Autodesk Inventor part; units mm, degrees
ref_plane "YZ Plane" through (0, 0, 0) normal (1, 0, 0) x (0, 1, 0)
ref_plane "XZ Plane" through (0, 0, 0) normal (0, 1, 0) x (-1, 0, 0)
ref_plane "XY Plane" through (0, 0, 0) normal (0, 0, 1) x (1, 0, 0)
sketch "Sketch1" plane through (0, 0, 0) normal (0, 0, 1) x (1, 0, 0)
  circle A0 centre (0, 0) radius 3.9624
  dimension "cap_diam" = 7.9248
extrude "Extrusion1" add sketch "Sketch1" along normal blind 4.826
sketch "Sketch2" plane through (0, 0, 0) normal (0, 0, -1) x (-1, 0, 0)
  circle A0 centre (0, 0) radius 3.9624
  circle A1 centre (0, 0) radius 2.413
  dimension "thread_diam" = 4.826
extrude "Extrusion2" add sketch "Sketch2" along normal blind 31.75 contours A1
thread "Thread1"
chamfer "Chamfer1" distance 0.4064 angle 45 1 edges at (2.413, 0, -31.75)
chamfer "Chamfer2" distance 0.635 angle 45 1 edges at (-3.9624, 0, 4.826)
sketch "Sketch4" plane through (0, 0, 4.826) normal (0, 0, 1) x (1, 0, 0)
  circle A0 centre (0, 0) radius 3.3274
  circle A1 centre (0, 0) radius 1.9844
  dimension "d21" = 3.9688
extrude "Extrusion4" cut sketch "Sketch4" against normal blind 0.3048 contours A1
chamfer "Chamfer3" distance 0.3048 angle 45 1 edges at (-1.9844, 0, 4.826)
sketch "Sketch5" plane through (0, 0, 4.826) normal (0, 0, 1) x (1, 0, 0)
  circle A0 centre (0, 0) radius 2.2892 construction
  line L0 (0, 2.2914) -> (1.9844, 1.1457)
  line L1 (1.9844, 1.1457) -> (1.9844, -1.1457)
  line L2 (1.9844, -1.1457) -> (0, -2.2914)
  line L3 (0, -2.2914) -> (-1.9844, -1.1457)
  line L4 (-1.9844, -1.1457) -> (-1.9844, 1.1457)
  line L5 (-1.9844, 1.1457) -> (0, 2.2914)
  dimension "d27" = 3.9688
extrude "Extrusion5" cut sketch "Sketch5" against normal blind 2.9718
equation "\"d21\" = hex_diam"
properties part number "10-32 x1000" material "Steel"
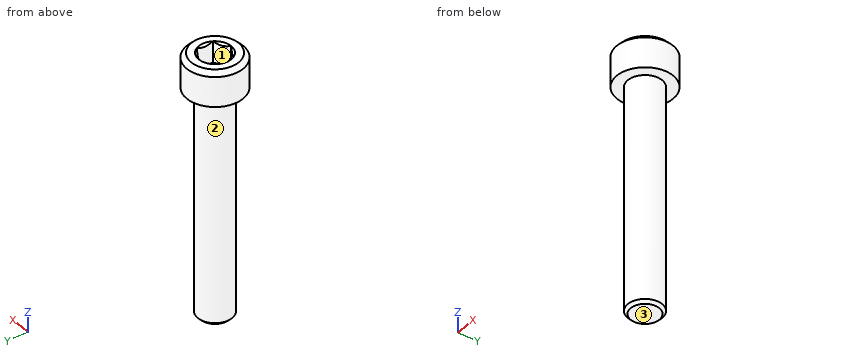
The model under review builds one solid part; all positions refer to its coordinate system, in mm. Face numbers are marked on the shaded views. Give positions to 0.01 mm unless a question says otherwise; leave off trailing zeros. Write each loop counter-clockwise with the first axis right and the second up, starting at its lowest first coordinate (ties: lowest second). Pieces come first, ordered by that corner, then holes. Notation, with made-up numbers: (39, -37.5) - (72, -37.5) arc R37 cw to (72, -1.5) - close; hole circle Ø8 at (35.25, -11.75). An arc over 180 degrees is marked (long way). Answer in a Markdown table with one row per item. Add a question column.
1. Draft analysis for pull direction X (two halves, no side actions). For the marked faces 1, 2 and 3, state which applies: +X half, -X half, draft (parallel to the pull), parting line (faces both ways), or undercut.
2. We need section A-A on y = 0. Write out the cut boundary in (x, z), then the cut area to 3 significant figures.
3. We need section B-B on z = -12.5. Write out the cut boundary in (x, y), then the cut area to 3 significant figures.
4. Wall thickness on line 1 along X through (y, z) = (1.5, 2.5); line 2 along Z through (x, y) = (-2.5, 1.5); line 3 along Z through (x, y) = (1.5, -1.25): over which ranges is each line inside the solid? List them lowest first. Write a range as [from, to].
5. Insertion check: P1, Ø1, axis at y = -1.5, z = -1, coming from the -X side; P2, Ø1.5, axis at x = -2.5, z = -1, coming from the -Y side; P3, Ø1, axis at y = 0.5, z = -20, coming from the +X side. Each pin has a flat end and moves straight along its axis. Give the tip position at first contact, or say it passes through.
Ans:
| question | item | result |
|---|---|---|
| 1 | face 1 | undercut |
| 1 | face 2 | parting line |
| 1 | face 3 | draft |
| 2 | outline | (-3.96, 0) - (-2.41, 0) - (-2.41, -31.34) - (-2.01, -31.75) - (2.01, -31.75) - (2.41, -31.34) - (2.41, 0) - (3.96, 0) - (3.96, 4.19) - (3.33, 4.83) - (2.29, 4.83) - (1.98, 4.52) - (1.98, 1.85) - (-1.98, 1.85) - (-1.98, 4.52) - (-2.29, 4.83) - (-3.33, 4.83) - (-3.96, 4.19) - close |
| 2 | area | 179 mm^2 |
| 3 | outline | circle Ø4.83 at (0, 0) |
| 3 | area | 18.3 mm^2 |
| 4 | line 1 | x = [-3.67, -1.37], [1.37, 3.67] |
| 4 | line 2 | z = [0, 4.83] |
| 4 | line 3 | z = [-31.75, 1.85] |
| 5 | P1 | stops at x = -2.2 |
| 5 | P2 | stops at y = -1.66 |
| 5 | P3 | stops at x = 2.41 |
